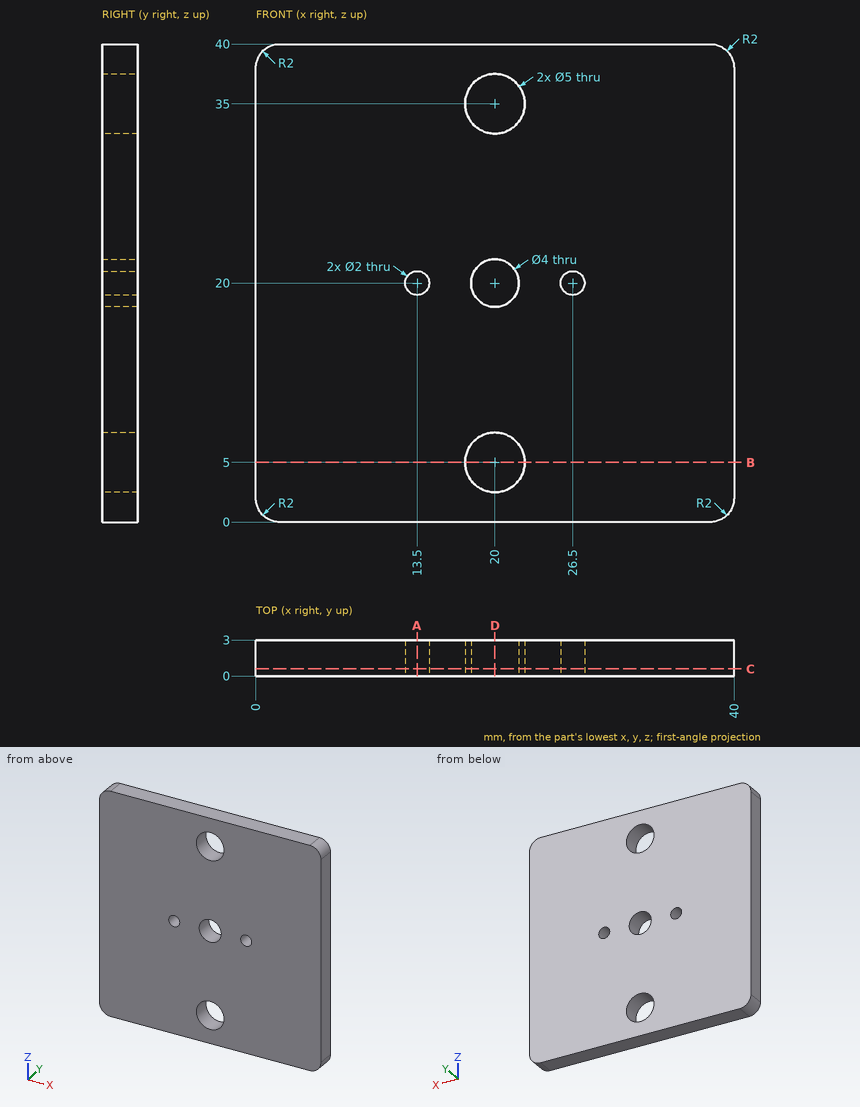
Source: three-view drawing plus pictorial views. Frame: mm from the lowest corner of the part. Round coordinates to 2 decimals unless told otherwise and drop trailing zeros. Order: outer loops, then holes, each group sorted by start corner. A loop starts at its lowest first (then second) coordinate and runs counter-clockwise, first axis right, second up. Notation, with made-up numbers: (-9, 9.25) -> (33, 9.25) arc R20 ccw to (33, 29.25) -> close; hole circle Ø8 at (21.25, 55). An arc over 180 degrees is marked (long way). Use one line per item in the form item = value.
(1) Ray query, probe 1 along Z at (x, y) = (20, 1.1); probe 2 along X at (y, z) = (2.2, 20); probe 3 along X at (y, z) = (2.1, 5). Return the intervals inside material, ascending. Write a range as [from, to].
Results list:
probe_1 = [0, 2.5], [7.5, 18], [22, 32.5], [37.5, 40]
probe_2 = [0, 12.5], [14.5, 18], [22, 25.5], [27.5, 40]
probe_3 = [0, 17.5], [22.5, 40]
(2) Section B-B on z = 5. Return loops of the section in (x, y).
Results list:
outline = (0, 0) -> (17.5, 0) -> (17.5, 3) -> (0, 3) -> close; (22.5, 0) -> (40, 0) -> (40, 3) -> (22.5, 3) -> close
(3) Section A-A on x = 13.5. Return loops of the section in (y, z), and give its area (3 significant figures).
Results list:
outline = (0, 0) -> (3, 0) -> (3, 19) -> (0, 19) -> close; (0, 21) -> (3, 21) -> (3, 40) -> (0, 40) -> close
area = 114 mm^2
(4) Section C-C on y = 0.6. Return loops of the section in (x, z).
Results list:
outline = (0, 2) arc R2 ccw to (2, 0) -> (38, 0) arc R2 ccw to (40, 2) -> (40, 38) arc R2 ccw to (38, 40) -> (2, 40) arc R2 ccw to (0, 38) -> close; hole circle Ø2 at (13.5, 20); hole circle Ø5 at (20, 5); hole circle Ø5 at (20, 35); hole circle Ø4 at (20, 20); hole circle Ø2 at (26.5, 20)
(5) Section D-D on x = 20. Return loops of the section in (y, z).
Results list:
outline = (0, 0) -> (3, 0) -> (3, 2.5) -> (0, 2.5) -> close; (0, 7.5) -> (3, 7.5) -> (3, 18) -> (0, 18) -> close; (0, 22) -> (3, 22) -> (3, 32.5) -> (0, 32.5) -> close; (0, 37.5) -> (3, 37.5) -> (3, 40) -> (0, 40) -> close
